Geometry: see drawing. Coordinates: mm, zero at the bounding-box minimum. A direction names the side the tool comes from. Round coordinates to 2 decimals unless told otherwise and drop trailing zeros. Loops run counter-clockwise (first coordinate to the right, second up) from the corner with the lowest first, then second, coordinate; pieces in that order, holes last. Notation, with made-up numbers: (48.25, 69.5) - (88.25, 69.5) arc R20 cw to (88.25, 80.5) - close; hole circle Ø9 at (-10.75, 49). An arc over 180 degrees is marked (long way). Use CSV: the item, a comma, the result in double quotes.
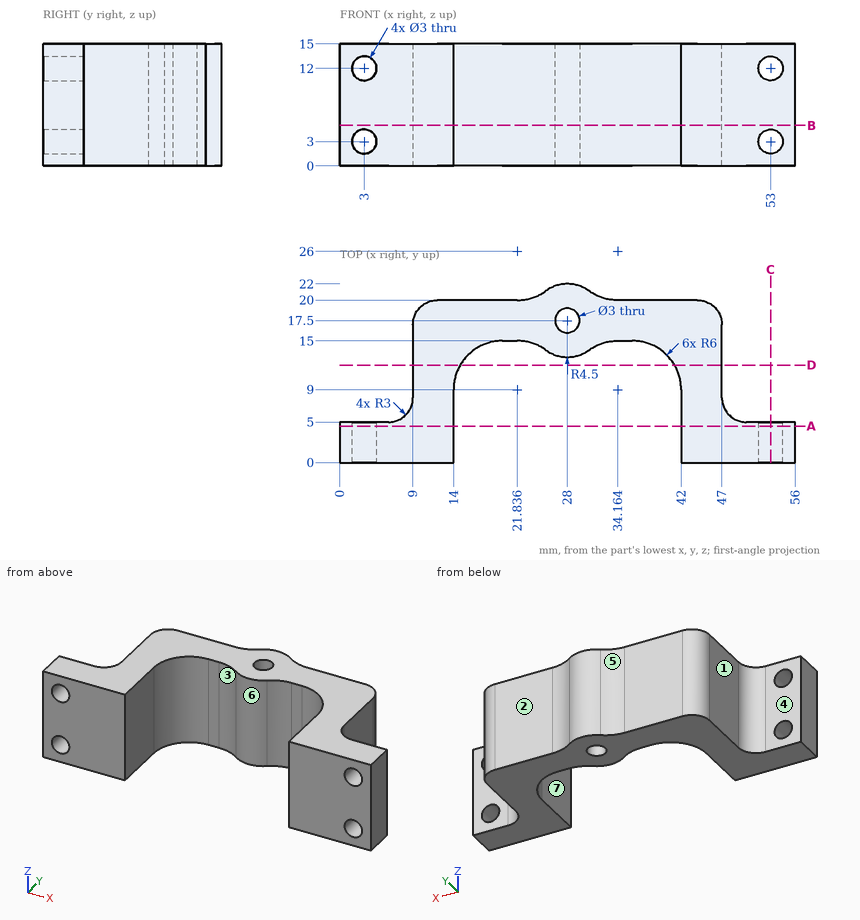
Item 1: Section C-C on x = 53. Return the cut outline in (y, z).
Final values:
outline,"(0, 0) - (5, 0) - (5, 1.5) - (0, 1.5) - close; (0, 4.5) - (5, 4.5) - (5, 10.5) - (0, 10.5) - close; (0, 13.5) - (5, 13.5) - (5, 15) - (0, 15) - close"
Item 2: Pin query (flat end, axial travel): P1, Ø3, axis at y = 16, z = 7, coming from the -X side; P2, Ø3, axis at x = 52, z = 8, coming from the +Y side; P3, Ø4.5, axis at y = 5, z = 6.5, coming from the -X side; P4, Ø2, axis at x = 20.5, z = 9.5, coming from the -Y side. Return the tip coordinate at first contact, or that it passes through.
Final values:
P1,"stops at x = 9"
P2,"stops at y = 5"
P3,"stops at x = 0"
P4,"stops at y = 14.98"
Item 3: Section D-D on y = 12. Return the cut outline in (x, z), plus the area to 3 significant figures.
Final values:
outline,"(9, 0) - (14.8, 0) - (14.8, 15) - (9, 15) - close; (41.2, 0) - (47, 0) - (47, 15) - (41.2, 15) - close"
area,"174 mm²"
Item 4: Section B-B on z = 5. Return the cut outline in (x, y) (1 decimal), plus the area to 3 significant figures.
Final values:
outline,"(0, 0) - (14, 0) - (14, 9) arc R6 cw to (20, 15) - (21.8, 15) arc R6 cw to (25.4, 13.9) arc R4.5 ccw to (30.6, 13.9) arc R6 cw to (34.2, 15) - (36, 15) arc R6 cw to (42, 9) - (42, 0) - (56, 0) - (56, 5) - (50, 5) arc R3 cw to (47, 8) - (47, 17) arc R3 ccw to (44, 20) - (34.2, 20) arc R6 cw to (30.6, 21.1) arc R4.5 ccw to (25.4, 21.1) arc R6 cw to (21.8, 20) - (12, 20) arc R3 ccw to (9, 17) - (9, 8) arc R3 cw to (6, 5) - (0, 5) - close; hole circle Ø3 at (28, 17.5)"
area,"462 mm²"
Item 5: Reachability of the marked faces 1, 2 and 3 from +Z, -Z, +X, -X, +Y, -Y: full face, straight path, thin tool, end or side. Return the list, or none.
Final values:
face 1,"+Z, -Z, -X, +Y"
face 2,"+Z, -Z, +X, +Y"
face 3,"+Z, -Z, -Y"
Item 6: Mould query, pull axis X, two halves, no side actions, for the marked faces 4, 5, 6 and 7. Classes: released by +X, released by -X, zero draft, split by the parting line, or undercut.
Final values:
face 4,"zero draft"
face 5,"released by -X"
face 6,"undercut"
face 7,"undercut"
Item 7: Section A-A on y = 4.5. Return the cut outline in (x, z), plus the area to 3 significant figures.
Final values:
outline,"(0, 0) - (14, 0) - (14, 15) - (0, 15) - close; (42, 0) - (56, 0) - (56, 15) - (42, 15) - close; hole circle Ø3 at (3, 3); hole circle Ø3 at (3, 12); hole circle Ø3 at (53, 3); hole circle Ø3 at (53, 12)"
area,"392 mm²"
Item 8: Material intervals for line 1 (Z direction, x = 3, y = 3.2); line 2 (Y direction, x = 12, z = 7.5); line 3 (X direction, y = 14.5, z = 5) (1 decimal), sorted ascending.
Final values:
line 1,"z = 0 to 1.5, 4.5 to 10.5, 13.5 to 15"
line 2,"y = 0 to 20"
line 3,"x = 9 to 17.6, 24.2 to 31.8, 38.4 to 47"
